Can you work these out from the drawing? Everything is in mm from the part's minimum corner. A direction names the side the tool comes from. Round coordinates to 2 decimals unless told otherwise and drop trailing zeros. Loops run counter-clockwise (first coordinate to the right, second up) from the corner with the lowest first, then second, coordinate; pieces in that order, holes last. Notation, with made-up numbers: M 64,17 L 123,17 A22 cw 123,34 Z; hole C 37,9 d4. An arc over 180 degrees is marked long. Use a Markdown table: item, result.
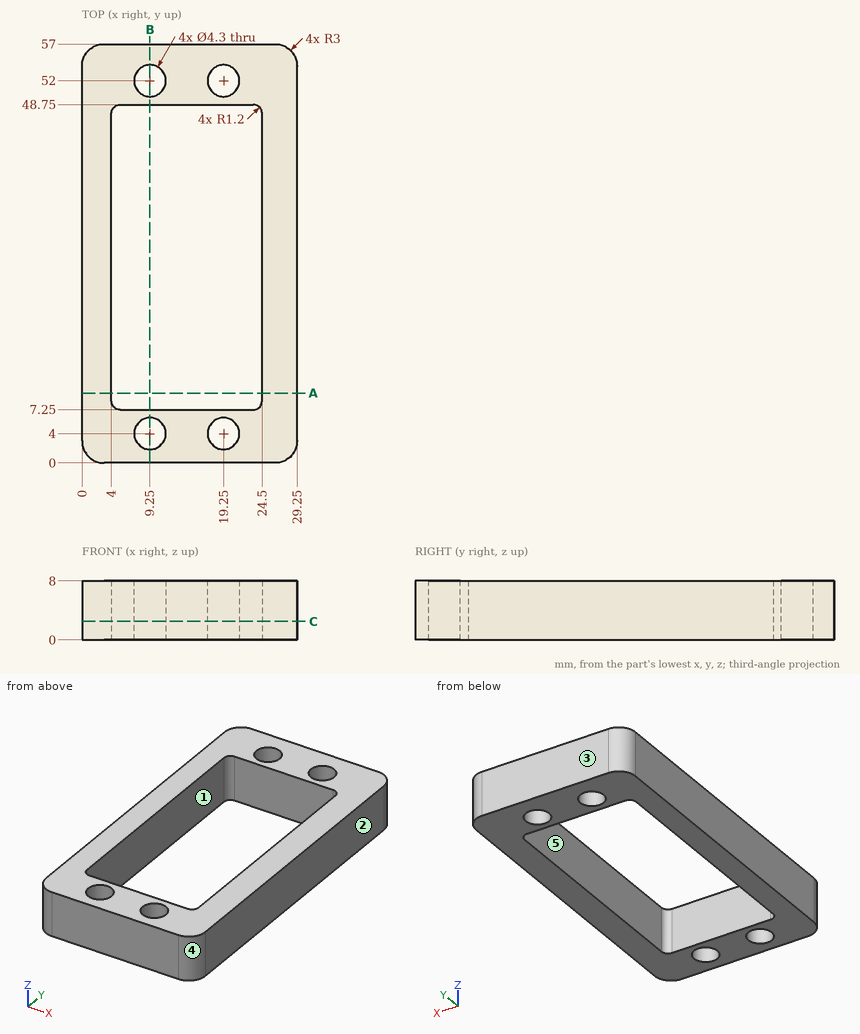
1. Imagine slicing it at C-C, the plane z = 2.5. Write out the boundary of the cut face in (x, y).
Answer sheet:
| item | result |
|---|---|
| outline | M 0,3 A3 ccw 3,0 L 26.25,0 A3 ccw 29.25,3 L 29.25,54 A3 ccw 26.25,57 L 3,57 A3 ccw 0,54 Z; hole M 4,8.45 A1.2 ccw 5.2,7.25 L 23.3,7.25 A1.2 ccw 24.5,8.45 L 24.5,47.55 A1.2 ccw 23.3,48.75 L 5.2,48.75 A1.2 ccw 4,47.55 Z; hole C 9.25,4 d4.3; hole C 9.25,52 d4.3; hole C 19.25,4 d4.3; hole C 19.25,52 d4.3 |
2. Imagine slicing it at B-B, the plane x = 9.25. Write out the boundary of the cut face in (y, z).
Answer sheet:
| item | result |
|---|---|
| outline | M 0,0 L 1.85,0 L 1.85,8 L 0,8 Z; M 6.15,0 L 7.25,0 L 7.25,8 L 6.15,8 Z; M 48.75,0 L 49.85,0 L 49.85,8 L 48.75,8 Z; M 54.15,0 L 57,0 L 57,8 L 54.15,8 Z |
3. I need wall thicknesses on probe 1 along Y at (x, z) = (19.25, 6.5); probe 2 along X at (y, z) = (18.5, 5.75); probe 3 along Y at (x, z) = (22.5, 6.25). Which ranges of each line are inside material? Lowest first, please. Write a range as from..to.
Answer sheet:
| item | result |
|---|---|
| probe 1 | 0..1.85, 6.15..7.25, 48.75..49.85, 54.15..57 |
| probe 2 | 0..4, 24.5..29.25 |
| probe 3 | 0..7.25, 48.75..57 |
4. Which directions (+Z, -Z, +X, -X, +Y, -Y) give clear straight access to the entire face, cutting with the end or side of a thin tool? Please do the marked faces 4 and 5.
Answer sheet:
| item | result |
|---|---|
| face 4 | +Z, -Z, +X, -Y |
| face 5 | +Z, -Z |
5. Imagine slicing it at A-A, the plane y = 9.5. Write out the boundary of the cut face in (x, z).
Answer sheet:
| item | result |
|---|---|
| outline | M 0,0 L 4,0 L 4,8 L 0,8 Z; M 24.5,0 L 29.25,0 L 29.25,8 L 24.5,8 Z |
6. For pin 1 Ø4 at (x, y) = (19.25, 52) entering from -Z; pin 2 Ø3 at (x, z) = (25.5, 3) entering from -Y, each with a flat end and sliding along its axis, tell me the tip position at first contact or that it passes through.
Answer sheet:
| item | result |
|---|---|
| pin 1 | through |
| pin 2 | y = 0 |
7. We'd pull the mould along X, two halves only. Please class the marked faces 1, 2 and 3: +X half, -X half, draft (parallel to the pull), parting line (faces both ways), or undercut.
Answer sheet:
| item | result |
|---|---|
| face 1 | undercut |
| face 2 | +X half |
| face 3 | draft |
